CAD build for the part. Positions are in the model's coordinates, mm. A direction names the side the tool comes from. Round coordinates to 2 decimals unless told otherwise and drop trailing zeros. Order: outer loops, then holes, each group sorted by start corner. A loop starts at its lowest first (then second) coordinate and runs counter-clockwise, first axis right, second up. Notation, with made-up numbers: (57.25, -28.5) -> (72.25, -28.5) arc R31 ccw to (72.25, 5.5) -> close; hole circle Ø8 at (-35, 23). An arc over 180 degrees is marked (long way). Return JSON: item names as keys, results as strings. Group by question number.
Q1. Probe line 1 along Y through (x, z) = (-1.25, 0.25); line 2 along Y through (x, z) = (0.5, -1); line 3 along Z through (x, y) = (-2, -1.75). List the from-to ranges inside material, lowest first.
Q2. Cut at C-C (y = -6.5). Write the cut outline in (x, z), then the cut area to 3 significant figures.
Q3. Mould opens along X. For faces 4 (the flat face through (1, 0, 0)), 5 (the cylindrical face through (2.97, -1.77, 0.94)), 6 (the flat face through (-0.75, -1, 0)) say: +X half, -X half, draft (parallel to the pull), parting line (faces both ways), or undercut.
Q4. Cut at D-D (y = -2.75). Write the cut outline in (x, z) (3 decimals).
Q5. Cut at B-B (x = 0). Write the cut outline in (y, z) (3 decimals), then the cut area to 3 significant figures.
Q6. Cut at A-A (z = 0). Write the cut outline in (x, y) (3 decimals), then the cut area to 3 significant figures.
Q7. Flat gauge pins, fed straight in: pin 1 (2 mm diameter, centred on x = -1.5, y = -6.5, fed in from -Z); pin 2 (1.5 mm diameter, centred on x = 1.5, y = -1.5, fed in from -Z); pin 3 (0.6 mm diameter, centred on y = -0.5, z = 1, fed in from -X). Where does each tip first touch, or does it go through?
Q8. Which spindle directions (+Z, -Z, +X, -X, +Y, -Y) get a long thin tool onto all of the face, cutting with end or side? Do faces 1 (the flat face through (0, -2, 0)), 2 (the flat face through (-1, -3, 1)), 3 (the flat face through (0, -10, 0)). Say none if no direction does.
from build123d import *

# Parameters (mm, degrees)
FILLET1_R          = 0.5
FILLET2_R          = 0.25
CUT_EXTRUDE1_DEPTH = 2


with BuildPart() as part:
    # Sketch2 → Revolve1 (revolve)
    with BuildSketch(Plane.XY):
        Polygon((0, 0), (3.115, 0), (3.115, -3), (0.99, -3), (0.99, -10), (0, -10), align=None)
    revolve(axis=Axis((0, 0, 0), (0, -1, 0)))

    # Fillet1
    fillet1_edges = [part.edges().sort_by_distance(p)[0] for p in [
        (-3.115, 0, 0),
    ]]
    fillet(fillet1_edges, radius=FILLET1_R)

    # Fillet2
    fillet2_edges = [part.edges().sort_by_distance(p)[0] for p in [
        (-0.99, -10, 0),
    ]]
    fillet(fillet2_edges, radius=FILLET2_R)

    # Sketch4 → Cut-Extrude1 (cut)
    with BuildSketch(Plane(origin=(0, 0, 0), x_dir=(1, 0, 0), z_dir=(0, 1, 0))):
        Polygon((0.75, -3), (0.75, 0.051459753), (0.75, 3), (-0.75, 3), (-0.75, -3), align=None)
    extrude(amount=-CUT_EXTRUDE1_DEPTH, mode=Mode.SUBTRACT)


solid = part.part
Solution:
{
 "1": {"line 1": "y = -3 to 0", "line 2": "y = -3 to -2", "line 3": "z = -2.39 to 2.39"},
 "2": {"outline": "circle Ø1.98 at (0, 0)", "area": "3.08 mm²"},
 "3": {"face 4": "draft", "face 5": "parting line", "face 6": "undercut"},
 "4": {"outline": "circle Ø6.23 at (0, 0)"},
 "5": {"outline": "(-10, -0.74) arc R0.25 ccw to (-9.75, -0.99) -> (-3, -0.99) -> (-3, -3.115) -> (-0.5, -3.115) arc R0.5 ccw to (-0.181, -3) -> (-2, -3) -> (-2, 3) -> (-0.181, 3) arc R0.5 ccw to (-0.5, 3.115) -> (-3, 3.115) -> (-3, 0.99) -> (-9.75, 0.99) arc R0.25 ccw to (-10, 0.74) -> close", "area": "20.5 mm²"},
 "6": {"outline": "(-3.115, -3) -> (-0.99, -3) -> (-0.99, -9.75) arc R0.25 ccw to (-0.74, -10) -> (0.74, -10) arc R0.25 ccw to (0.99, -9.75) -> (0.99, -3) -> (3.115, -3) -> (3.115, -0.5) arc R0.5 ccw to (2.615, 0) -> (0.75, 0) -> (0.75, -2) -> (-0.75, -2) -> (-0.75, 0) -> (-2.615, 0) arc R0.5 ccw to (-3.115, -0.5) -> close", "area": "29.4 mm²"},
 "7": {"pin 1": "stops at z = -0.85", "pin 2": "stops at z = -3.02", "pin 3": "stops at x = -3.04"},
 "8": {"face 1": "+Y", "face 2": "-Y", "face 3": "+Z, -Z, +X, -X, -Y"}
}
